Source: CAD feature listing. Evaluate the final solid. Frame: model axes, mm. A direction names the side the tool comes from. Give positions to 0.01 mm unless a question says otherwise; leave off trailing zeros. Write each loop counter-clockwise with the first axis right and the second up, starting at its lowest first coordinate (ties: lowest second). Pieces come first, ordered by that corner, then holes. Notation, with made-up numbers: (74, 0) -> (89, 0) arc R17 cw to (89, 15) -> close; hole circle Ø10 at (-4.5, 8). An arc over 180 degrees is marked (long way). Answer as a JSON object with one key per item and string values. Group by question number.
Item 1: Section query D-D on y = 18.25. Return the cut outline in (x, z), plus the area to 3 significant figures.
Item 2: Access query for faces 4 (the face through (-1.11, 6.01, -3.22)), 5 (the face through (2, 0, 0)), 6 (the face through (0, 16, 2)). Directions: +Z, -Z, +X, -X, +Y, -Y. A direction counts if a zero-diameter tool reaches every point of the face in a straight line with its end or side. Return the directions, or none.
Item 3: Section query A-A on z = 0. Return the cut outline in (x, y) (3 decimals).
Item 4: Section query C-C on x = 1. Give the number of separate pieces and of enclosed holes in the cut face, plus the area to 3 significant figures.
Item 5: Ray query, probe 1 along Y at (x, z) = (0, -2.45); probe 2 along Y at (x, z) = (0, -4.1); probe 3 along Z at (x, y) = (0, 5.5) (3 decimals). Return the intervals inside material, ascending. Write a range as from..to.
Item 6: First-contact query: pin 1 Ø3 at (x, y) = (3.5, 3.5) entering from +Z; pin 2 Ø1.9 at (x, z) = (0, 0) entering from +Y; pin 3 Ø4.5 at (x, z) = (0, 0) entering from +Y; pin 4 Ø1 at (y, z) = (17.5, -1) entering from +X. Flat tips, straight axial feed; report the tip coordinate or a pass-through.
Item 7: Pull-direction query (Z, two-part tool) for faces 1 (the face through (-0.34, 5.58, 1.55)), 2 (the face through (-1.08, 11.14, 4.88)), 3 (the face through (2, 22, -2)); classes: pulls with the +Z half, pulls with the -Z half, needs draft (parallel to the pull), parting line crosses it, or undercut.
Item 8: Section query B-B on y = 13.5. Return the cut outline in (x, z).
Autodesk Inventor part; units mm, degrees
ref_plane "YZ Plane" through (0, 0, 0) normal (1, 0, 0) x (0, 1, 0)
ref_plane "XZ Plane" through (0, 0, 0) normal (0, 1, 0) x (-1, 0, 0)
ref_plane "XY Plane" through (0, 0, 0) normal (0, 0, 1) x (1, 0, 0)
sketch "Sketch1" plane through (0, 0, 0) normal (0, 0, 1) x (1, 0, 0)
  line L0 (0, 0) -> (5, 0)
  line L1 (5, 0) -> (5, 22)
  line L2 (5, 22) -> (0, 22)
  line L3 (0, 0) -> (1.585, 0)
  line L4 (1.585, 0) -> (1.585, 11)
  line L5 (0, 22) -> (2, 22)
  line L6 (2, 22) -> (2, 11)
  line L7 (2, 11) -> (1.585, 11)
  circle A0 centre (0, 17) radius 1.5
  circle A1 centre (0, 5) radius 1.5
  line L8 (0, 0) -> (0, -2.0166)
  dimension "d0" = 5
  dimension "d1" = 22
  dimension "d2" = 1.585
  dimension "d3" = 2
  dimension "d4" = 3
  dimension "d5" = 3
  dimension "d6" = 5
  dimension "d7" = 5
revolve "Revolution1" add sketch "Sketch1" angle 360 about axis through (0, 0, 0) along (0, -1, 0) contours L4 L7 L6 L2 L1 L0
extrude "Extrusion1" cut sketch "Sketch1" against normal blind 25.4 contours A0 | A1
chamfer "Chamfer1" distance 1.27 angle 45 2 edges at (-5, 22, 0) (-5, 0, 0)
properties part number "MotorShaftCoupler"
Worked answers:
{
 "1": {"outline": "(-0.83, -4.93) -> (-0.83, -1.82) arc R2 cw (long way) to (0.83, -1.82) -> (0.83, -4.93) arc R5 ccw (long way) to start", "area": "60.9 mm^2"},
 "2": {"face 4": "-Z", "face 5": "+Z, -Z, +X, -X, -Y", "face 6": "+Y"},
 "3": {"outline": "(-5, 1.27) -> (-3.73, 0) -> (-1.585, 0) -> (-1.585, 11) -> (-2, 11) -> (-2, 22) -> (-3.73, 22) -> (-5, 20.73) -> close; (1.585, 0) -> (3.73, 0) -> (5, 1.27) -> (5, 20.73) -> (3.73, 22) -> (2, 22) -> (2, 11) -> (1.585, 11) -> close"},
 "4": {"separate pieces": "4", "enclosed holes": "0", "area": "132 mm^2"},
 "5": {"probe 1": "0..3.5, 6.5..15.5, 18.5..22", "probe 2": "0.37..3.5, 6.5..15.5, 18.5..21.63", "probe 3": "1.585..5"},
 "6": {"pin 1": "z = 4.58", "pin 2": "through", "pin 3": "y = 22", "pin 4": "x = 4.97"},
 "7": {"face 1": "undercut", "face 2": "parting line crosses it", "face 3": "needs draft"},
 "8": {"outline": "circle Ø10 at (0, 0); hole circle Ø4 at (0, 0)"}
}
